Here's how the part is built. I have some questions about the finished solid (model axes, mm). Coordinates: 2 decimals unless noted, no trailing zeros. Write each loop counter-clockwise with the first axis right and the second up, starting at its lowest first coordinate (ties: lowest second). Pieces come first, ordered by that corner, then holes.
(1) Imagine slicing it at C-C, the plane z = -14. List the corners of the cut face in (x, y) for me.
(2) Imagine slicing it at B-B, the plane x = 17. List the corners of the cut face in (y, z) for me.
(3) Please list where these lines run through material, in increasing order: probe 1 along Z at (x, y) = (17, 0.5); probe 2 along X at (y, z) = (0.4, -15); probe 3 along Z at (x, y) = (17.5, 0.45).
(4) For pin 1 Ø3 at (x, z) = (17, 15) entering from -Y, with a flat end and sliding along its axis, tell me the tip position at first contact or that it passes through.
(5) Imagine slicing it at A-A, the plane z = 15. List the corners of the cut face in (x, y) for me.
```python
from build123d import *

# Parameters (mm, degrees)
SKETCH1_W           = 39
SKETCH1_H           = 35
BOSS_EXTRUDE1_DEPTH = 1.6
CUT_EXTRUDE1_REACH  = 3.6
SKETCH2_R           = 1.6
FILLET1_R           = 1.6


with BuildPart() as part:
    # Sketch1 → Boss-Extrude1 (new body)
    with BuildSketch(Plane(origin=(0, 0, 0), x_dir=(1, 0, 0), z_dir=(0, 1, 0))):
        Rectangle(SKETCH1_W, SKETCH1_H)
    extrude(amount=BOSS_EXTRUDE1_DEPTH)

    # Sketch2 → Cut-Extrude1 (cut, up to next)
    with BuildSketch(Plane(origin=(0, 1.6, 0), x_dir=(1, 0, 0), z_dir=(0, 1, 0)), mode=Mode.PRIVATE) as cut_extrude1_sk1:
        with Locations((17, 15)):
            Circle(SKETCH2_R)
    cut_extrude1_tool1 = extrude(cut_extrude1_sk1.sketch, amount=-CUT_EXTRUDE1_REACH, mode=Mode.PRIVATE) & part.part
    add(cut_extrude1_tool1.solids().sort_by_distance((17, 1.6, -15))[0], mode=Mode.SUBTRACT)
    # Sketch2 → Cut-Extrude1 (cut, up to next)
    with BuildSketch(Plane(origin=(0, 1.6, 0), x_dir=(1, 0, 0), z_dir=(0, 1, 0)), mode=Mode.PRIVATE) as cut_extrude1_sk2:
        with Locations((17, -15)):
            Circle(SKETCH2_R)
    cut_extrude1_tool2 = extrude(cut_extrude1_sk2.sketch, amount=-CUT_EXTRUDE1_REACH, mode=Mode.PRIVATE) & part.part
    add(cut_extrude1_tool2.solids().sort_by_distance((17, 1.6, 15))[0], mode=Mode.SUBTRACT)

    # Fillet1
    fillet1_edges = [part.edges().sort_by_distance(p)[0] for p in [
        (19.5, 0.8, 17.5),
        (19.5, 0.8, -17.5),
    ]]
    fillet(fillet1_edges, radius=FILLET1_R)


solid = part.part
```
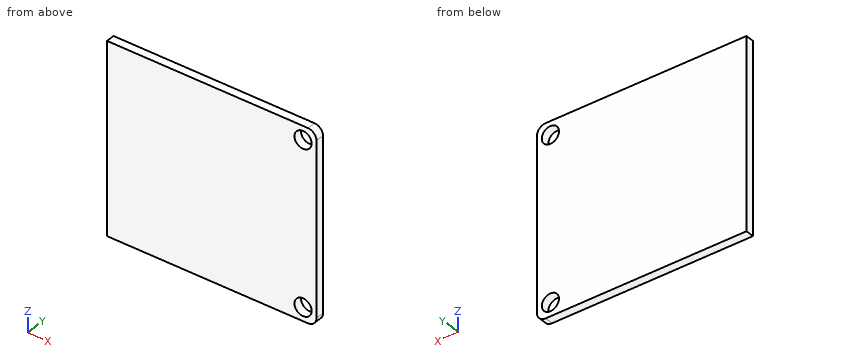
Recorded:
1. outline: (-19.5, 0) - (15.75, 0) - (15.75, 1.6) - (-19.5, 1.6) - close; (18.25, 0) - (19.5, 0) - (19.5, 1.6) - (18.25, 1.6) - close
2. outline: (0, -17.5) - (1.6, -17.5) - (1.6, -16.6) - (0, -16.6) - close; (0, -13.4) - (1.6, -13.4) - (1.6, 13.4) - (0, 13.4) - close; (0, 16.6) - (1.6, 16.6) - (1.6, 17.5) - (0, 17.5) - close
3. probe 1: z = -17.5 to -16.6, -13.4 to 13.4, 16.6 to 17.5
3. probe 2: x = -19.5 to 15.4, 18.6 to 19.5
3. probe 3: z = -17.5 to -16.52, -13.48 to 13.48, 16.52 to 17.5
4. pin 1: passes through
5. outline: (-19.5, 0) - (15.4, 0) - (15.4, 1.6) - (-19.5, 1.6) - close; (18.6, 0) - (19.5, 0) - (19.5, 1.6) - (18.6, 1.6) - close
